For this review, take the finished solid that the model builds, in its own axes (mm). Give positions to 0.01 mm unless a question says otherwise; leave off trailing zeros. Write each loop counter-clockwise with the first axis right and the second up, starting at its lowest first coordinate (ties: lowest second). Pieces come first, ordered by that corner, then holes. Notation, with made-up numbers: (18.5, -8.5) -> (62.5, -8.5) arc R11 cw to (62.5, 0.5) -> close; hole circle Ø2 at (35, 18). An arc over 180 degrees is marked (long way). Return JSON: item names as keys, results as strings.
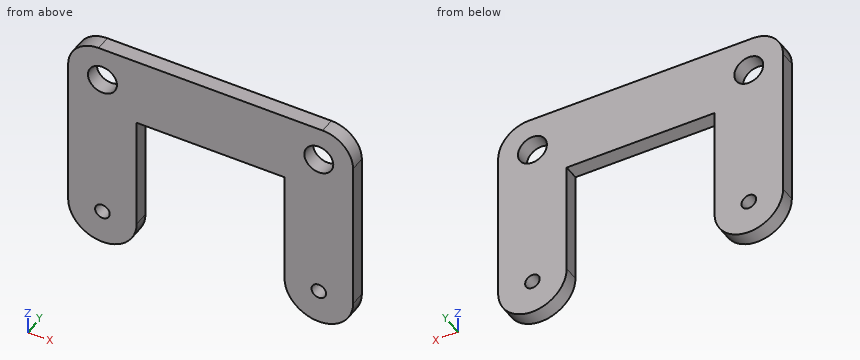
from build123d import *

# Parameters (mm, degrees)
SKETCH1_R           = 4.75
SKETCH1_R_2         = 11.25
SKETCH1_R_3         = 2.4
BOSS_EXTRUDE1_DEPTH = 5
FILLET1_R           = 10


with BuildPart() as part:
    # Sketch1 → Boss-Extrude1 (new body)
    with BuildSketch(Plane(origin=(0, 0, 0), x_dir=(1, 0, 0), z_dir=(0, 1, 0))):
        with BuildLine():
            Line((-24.25, -37.5), (-24.25, 0))
            ThreePointArc((-24.25, 0), (-35.5, -11.25), (-46.75, 0))
            Line((-46.75, 0), (-46.75, -60))
            Line((-46.75, -60), (46.75, -60))
            Line((46.75, -60), (46.75, 0))
            ThreePointArc((46.75, 0), (35.5, -11.25), (24.25, 0))
            Line((24.25, 0), (24.25, -37.5))
            Line((24.25, -37.5), (-24.25, -37.5))
        make_face()
        with Locations((-35.5, -48.75)):
            Circle(SKETCH1_R, mode=Mode.SUBTRACT)
        with Locations((35.5, -48.75)):
            Circle(SKETCH1_R, mode=Mode.SUBTRACT)
        with Locations((-35.5, 0)):
            Circle(SKETCH1_R_2)
        with Locations((-35.5, 0)):
            Circle(SKETCH1_R_3, mode=Mode.SUBTRACT)
        with Locations((35.5, 0)):
            Circle(SKETCH1_R_2)
        with Locations((35.5, 0)):
            Circle(SKETCH1_R_3, mode=Mode.SUBTRACT)
    extrude(amount=BOSS_EXTRUDE1_DEPTH)

    # Fillet1
    fillet1_edges = [part.edges().sort_by_distance(p)[0] for p in [
        (46.75, 2.5, 60),
        (-46.75, 2.5, 60),
    ]]
    fillet(fillet1_edges, radius=FILLET1_R)


solid = part.part
1. For pin 1 (3 mm diameter, centred on x = 22.5, y = 3.5, fed in from -Z), flat-tipped, find the tip position at first contact; note if it passes through.
Results found:
{"pin 1": "stops at z = 37.5"}
2. Add section B-B, the plane z = 48.75. State the section outline as (x, y) points, plus the area to 4 significant figures.
Results found:
{"outline": "(-46.75, 0) -> (-40.25, 0) -> (-40.25, 5) -> (-46.75, 5) -> close; (-30.75, 0) -> (30.75, 0) -> (30.75, 5) -> (-30.75, 5) -> close; (40.25, 0) -> (46.75, 0) -> (46.75, 5) -> (40.25, 5) -> close", "area": "372.5 mm²"}
3. Add section D-D, the plane z = 25. State the section outline as (x, y) points, plus the area to 3 significant figures.
Results found:
{"outline": "(-46.75, 0) -> (-24.25, 0) -> (-24.25, 5) -> (-46.75, 5) -> close; (24.25, 0) -> (46.75, 0) -> (46.75, 5) -> (24.25, 5) -> close", "area": "225 mm²"}
4. Add section A-A, the plane x = -35.5. State the section outline as (y, z) points.
Results found:
{"outline": "(0, -11.25) -> (5, -11.25) -> (5, -2.4) -> (0, -2.4) -> close; (0, 2.4) -> (5, 2.4) -> (5, 44) -> (0, 44) -> close; (0, 53.5) -> (5, 53.5) -> (5, 60) -> (0, 60) -> close"}
5. To check wall thickness, follow probe 1 along X at (y, z) = (2.45, 48.75); probe 2 along Z at (x, y) = (-35.5, 3.25); probe 3 along X at (y, z) = (0.55, 3). State the ranges of each line that lie inside material, in increasing order.
Results found:
{"probe 1": "x = -46.75 to -40.25, -30.75 to 30.75, 40.25 to 46.75", "probe 2": "z = -11.25 to -2.4, 2.4 to 44, 53.5 to 60", "probe 3": "x = -46.75 to -24.25, 24.25 to 46.75"}
6. Add section C-C, the plane y = 0.9. State the section outline as (x, z) points.
Results found:
{"outline": "(-46.75, 0) arc R11.25 ccw to (-24.25, 0) -> (-24.25, 37.5) -> (24.25, 37.5) -> (24.25, 0) arc R11.25 ccw to (46.75, 0) -> (46.75, 50) arc R10 ccw to (36.75, 60) -> (-36.75, 60) arc R10 ccw to (-46.75, 50) -> close; hole circle Ø9.5 at (-35.5, 48.75); hole circle Ø4.8 at (-35.5, 0); hole circle Ø9.5 at (35.5, 48.75); hole circle Ø4.8 at (35.5, 0)"}
